Part model, mm, in its own coordinate system. Face numbers are marked on the shaded views. A direction names the side the tool comes from. Give positions to 0.01 mm unless a question says otherwise; leave off trailing zeros. Loops run counter-clockwise (first coordinate to the right, second up) from the corner with the lowest first, then second, coordinate; pieces in that order, holes last. Notation, with made-up numbers: M -11.75,-20 L 6.25,-20 A15 cw 6.25,-2 Z; hole C 75.5,-29.5 d7. An arc over 180 degrees is marked long. Put each result on its own line as item: value. Start each with the question number.
```python
from build123d import *

# Parameters (mm, degrees)
BOSS_EXTRUDE1_DEPTH     = 60
CUT_EXTRUDE1_DEPTH      = 104.638795825
CUT_EXTRUDE1_DEPTH_BACK = 104.638795825
BOSS_EXTRUDE2_DEPTH     = 10
SKETCH5_R               = 10
CUT_EXTRUDE2_DEPTH      = 93.200867675


with BuildPart() as part:
    # Sketch1 → Boss-Extrude1 (new body)
    with BuildSketch(Plane.XY):
        Polygon((-30, 30), (-49, 0), (-18, 0), (-18, 10), (0, 10), (0, 30), (-20, 30), align=None)
        Polygon((20, 30), (0, 30), (0, 10), (18, 10), (18, 0), (49, 0), (30, 30), align=None)
    extrude(amount=-BOSS_EXTRUDE1_DEPTH)

    # Sketch3 → Cut-Extrude1 (cut, two sides: drawn at the far end of the back side and taken through both)
    with BuildSketch(Plane(origin=(30, 0, 0), x_dir=(0, 0, -1), z_dir=(1, 0, 0)).offset(-CUT_EXTRUDE1_DEPTH_BACK)):
        Polygon((17, 144.861813831), (17, 30), (17, 19.936985668), (43, 19.936985668), (43, 30), (43, 144.861813831), (43, 374.585441494), (17, 374.585441494), align=None)
    extrude(amount=CUT_EXTRUDE1_DEPTH + CUT_EXTRUDE1_DEPTH_BACK, mode=Mode.SUBTRACT)

    # Sketch4 → Boss-Extrude2 (add)
    with BuildSketch(Plane.XY):
        with BuildLine():
            Line((-20, 30), (20, 30))
            ThreePointArc((20, 30), (0, 50), (-20, 30))
        make_face()
    boss_extrude2 = extrude(amount=-BOSS_EXTRUDE2_DEPTH)

    # Sketch5 → Cut-Extrude2 (cut, through all)
    with BuildSketch(Plane.XY):
        with Locations((0, 30)):
            Circle(SKETCH5_R)
    cut_extrude2 = extrude(amount=-CUT_EXTRUDE2_DEPTH, mode=Mode.SUBTRACT)

    # Mirror1: Boss-Extrude2 across plane
    add(boss_extrude2.mirror(Plane.XY.offset(-30)))

    # Mirror2: Cut-Extrude2 across plane
    add(cut_extrude2.mirror(Plane.XY.offset(-30)), mode=Mode.SUBTRACT)


solid = part.part
```
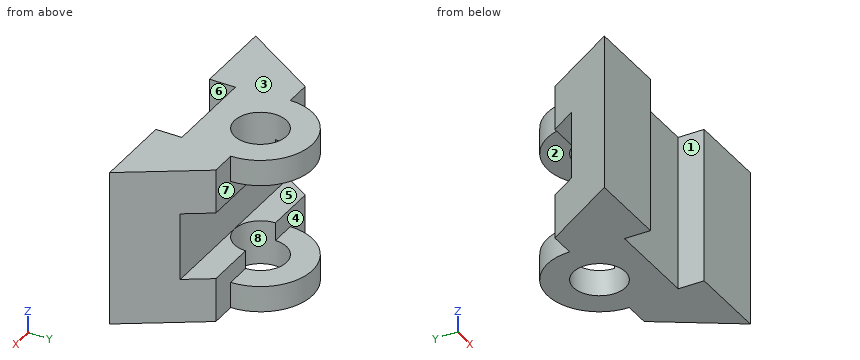
1) Pin check, flat tips, straight feed: pin 1 Ø8.5 at (x, z) = (24.5, -6.5) entering from +Y; pin 2 Ø8 at (x, z) = (35.5, -12.5) entering from -Y; pin 3 Ø13.5 at (x, z) = (-22, -54.5) entering from +Y; pin 4 Ø12 at (y, z) = (18.5, -17.5) entering from -X. Stop position of each tip, or through.
2) Which spindle directions (+Z, -Z, +X, -X, +Y, -Y) get a long thin tool onto all of the face, cutting with end or side? Do the marked faces 4, 5, 6, 7 and 8. Say none if no direction does.
3) Band-saw the part on D-D on y = 4.5. Give the cut face in (x, z).
4) Band-saw the part on C-C on z = -18.5. Give the cut face in (x, y), then the cut area to 3 significant figures.
5) Wall check: L1, parallel to Z at x = -21, y = 29; L2, parallel to Y at x = 0, z = -54; L3, parallel to Y at x = -25, z = -20.5. Give the ranges that are in metal, low to high.
6) Band-saw the part on A-A on y = 24. Give the cut face in (x, z).
7) Band-saw the part on B-B on x = 0. Give the cut face in (y, z), then the cut area to 3 significant figures.
8) Mould opens along Z. For the marked faces 1, 2 and 3 say: +Z half, -Z half, draft (parallel to the pull), parting line (faces both ways), or undercut.
Evaluation:
1. pin 1: y = 30
1. pin 2: y = 0
1. pin 3: y = 42.94
1. pin 4: x = -41.08
2. face 4: -X, +Y
2. face 5: +X, -X, +Y
2. face 6: +Z, -Z, -Y
2. face 7: +X, +Y
2. face 8: +Z, -Z
3. outline: M -46.15,-60 L -18,-60 L -18,0 L -46.15,0 Z; M 18,-60 L 46.15,-60 L 46.15,0 L 18,0 Z
4. outline: M -49,0 L -18,0 L -18,10 L 18,10 L 18,0 L 49,0 L 36.37,19.94 L -36.37,19.94 Z
4. area: 1,340 mm2
5. L1: -60 to -43, -17 to 0
5. L2: 10 to 20, 40 to 50
5. L3: 0 to 19.94
6. outline: M -33.8,-60 L -8,-60 L -8,-43 L -33.8,-43 Z; M -33.8,-17 L -8,-17 L -8,0 L -33.8,0 Z; M 8,-60 L 33.8,-60 L 33.8,-43 L 8,-43 Z; M 8,-17 L 33.8,-17 L 33.8,0 L 8,0 Z
7. outline: M 10,-60 L 20,-60 L 20,-43 L 19.94,-43 L 19.94,-17 L 20,-17 L 20,0 L 10,0 Z; M 40,-60 L 50,-60 L 50,-50 L 40,-50 Z; M 40,-10 L 50,-10 L 50,0 L 40,0 Z
7. area: 798 mm2
8. face 1: draft
8. face 2: undercut
8. face 3: +Z half
